For this review, use the dimensioned drawing (mm, ordinates from the lowest corner) and the shaded views. Coordinates: 2 decimals unless noted, no trailing zeros. Loops run counter-clockwise (first coordinate to the right, second up) from the corner with the lowest first, then second, coordinate; pieces in that order, holes last. Notation, with made-up numbers: (19, -20.75) -> (70, -20.75) arc R16 ccw to (70, -11.75) -> close; hole circle Ø2 at (74.5, 18.5). An arc over 180 degrees is marked (long way). One line per question, with ' | ' between items. Start each with the question number.
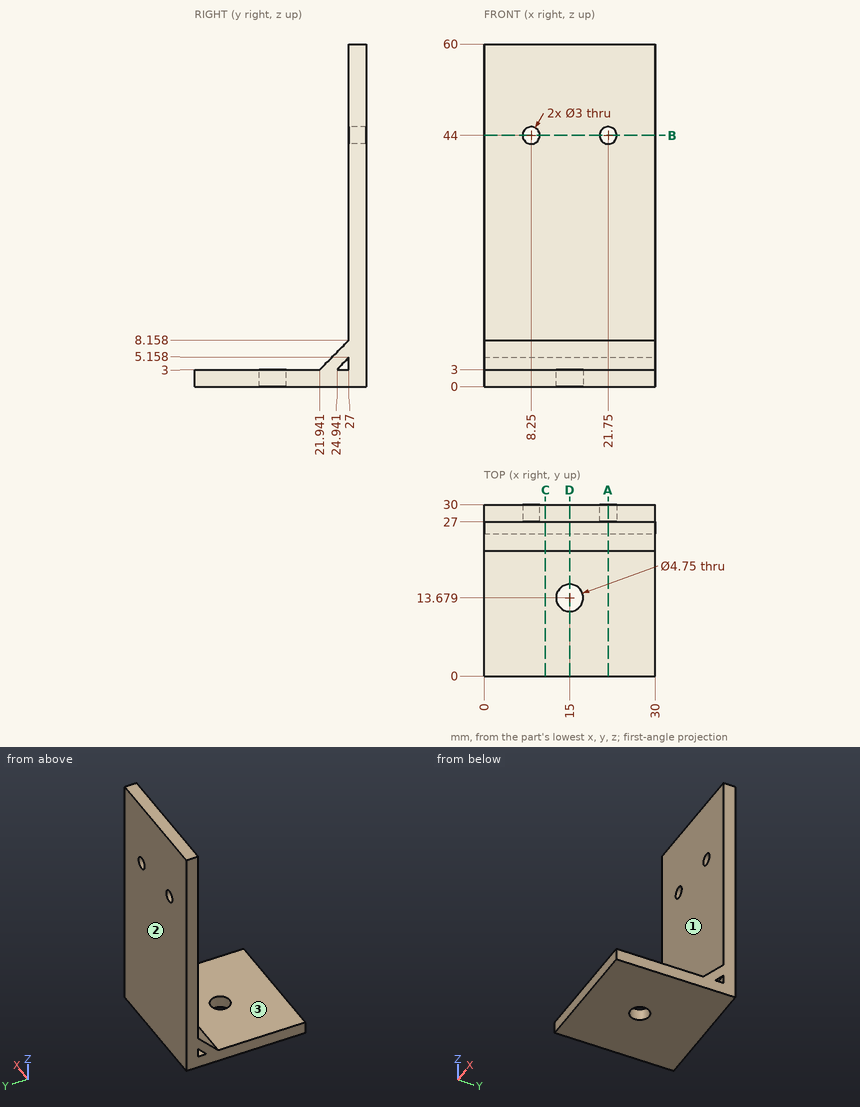
1) Mouldability with a two-part tool opening along Y and no side actions: class the marked faces 1, 2 and 3 as +Y half, -Y half, draft (parallel to the pull), parting line (faces both ways), or undercut.
2) Wall thickness on L1, parallel to Z at x = 8.25, y = 29.1; L2, parallel to Y at x = 15, z = 1.4; L3, parallel to Z at x = 11, y = 20: over which ranges is each line inside the solid? List them lowest first.
3) Consider section B-B, the plane z = 44. Write out the cut boundary in (x, y).
4) Insertion check: pin 1 Ø2.5 at (x, z) = (8.25, 44) entering from -Y; pin 2 Ø1.5 at (x, z) = (6.5, 18) entering from -Y; pin 3 Ø17.5 at (x, y) = (8.5, 6.5) entering from +Z. Each pin has a flat end and moves straight along its axis. Give the tip position at first contact, or say it passes through.
5) Consider section C-C, the plane x = 10.75. Write out the cut boundary in (y, z), plus the area to 3 significant figures.
6) Consider section A-A, the plane x = 21.75. Write out the cut boundary in (y, z).
7) Consider section D-D, the plane x = 15. Write out the cut boundary in (y, z).
Filled sheet:
1) face 1: -Y half | face 2: +Y half | face 3: draft
2) L1: 0 to 42.5, 45.5 to 60 | L2: 0 to 11.3, 16.05 to 30 | L3: 0 to 3
3) outline: (0, 27) -> (6.75, 27) -> (6.75, 30) -> (0, 30) -> close; (9.75, 27) -> (20.25, 27) -> (20.25, 30) -> (9.75, 30) -> close; (23.25, 27) -> (30, 27) -> (30, 30) -> (23.25, 30) -> close
4) pin 1: through | pin 2: y = 27 | pin 3: z = 3
5) outline: (0, 0) -> (30, 0) -> (30, 60) -> (27, 60) -> (27, 8.16) -> (21.94, 3) -> (0, 3) -> close; hole (24.94, 3) -> (27, 3) -> (27, 5.16) -> close | area: 272 mm^2
6) outline: (0, 0) -> (30, 0) -> (30, 42.5) -> (27, 42.5) -> (27, 8.16) -> (21.94, 3) -> (0, 3) -> close; (27, 45.5) -> (30, 45.5) -> (30, 60) -> (27, 60) -> close; hole (24.94, 3) -> (27, 3) -> (27, 5.16) -> close
7) outline: (0, 0) -> (11.3, 0) -> (11.3, 3) -> (0, 3) -> close; (16.05, 0) -> (30, 0) -> (30, 60) -> (27, 60) -> (27, 8.16) -> (21.94, 3) -> (16.05, 3) -> close; hole (24.94, 3) -> (27, 3) -> (27, 5.16) -> close
